```python
from build123d import *

# Parameters (mm, degrees)
BOSS_EXTRUDE1_DEPTH = 30
SKETCH2_R           = 2.5
CUT_EXTRUDE1_DEPTH  = 30


with BuildPart() as part:
    # Sketch1 → Boss-Extrude1 (new body)
    with BuildSketch(Plane.XY):
        with BuildLine():
            Line((0, 50), (0, 0))
            ThreePointArc((0, 0), (59.137285401, -30.145421821), (82.921098745, -92.115537233))
            Line((82.921098745, -92.115537233), (82.921098745, -120))
            Line((82.921098745, -120), (85.921098745, -120))
            Line((85.921098745, -120), (85.921098745, -92.115537233))
            ThreePointArc((85.921098745, -92.115537233), (62.264683971, -29.149857277), (3, 2.662090888))
            Line((3, 2.662090888), (3, 50))
            Line((3, 50), (0, 50))
        make_face()
    extrude(amount=BOSS_EXTRUDE1_DEPTH)

    # Sketch2 → Cut-Extrude1 (cut)
    with BuildSketch(Plane(origin=(85.921098745, 0, 0), x_dir=(0, 0, -1), z_dir=(1, 0, 0))):
        with Locations(Location((-15, -106.057768617, 0), (0, 0, 90))):
            Circle(SKETCH2_R)
    extrude(amount=-CUT_EXTRUDE1_DEPTH, mode=Mode.SUBTRACT)


solid = part.part
```
The model under review builds one solid part; all positions refer to its coordinate system, in mm. A direction names the side the tool comes from. Give positions to 0.01 mm unless a question says otherwise; leave off trailing zeros. Write each loop counter-clockwise with the first axis right and the second up, starting at its lowest first coordinate (ties: lowest second). Pieces come first, ordered by that corner, then holes. Notation, with made-up numbers: M 2.25,46.5 L 60.25,46.5 A17 cw 60.25,79.5 Z; hole C 15,-34 d9. An arc over 180 degrees is marked long. Write item = value, one per line. Start each with the question number.
Q1. For line 1 (X direction, y = 31, z = 6.25); line 2 (X direction, y = -107, z = 17.5); line 3 (Y direction, x = 27.5, z = 4.75), list the stretches that pass through material, from the lowest coordinate up.
Q2. We need section C-C (y = 38.5). State the section outline as (x, z) points, plus the area to 3 significant figures.
Q3. Machinability: for faces 1 (the face through (84, -120, 15)), 2 (the face through (3, 26, 15)), which of the approach directions +Z, -Z, +X, -X, +Y, -Y give a long, thin tool a straight path to every point of the face, cutting with its end or side? Answer none if there is none.
Q4. Mouldability with a two-part tool opening along Y and no side actions: class faces 3 (the face through (82.921, -103, 15)), 4 (the face through (84.442, -104.904, 12.782)), 5 (the face through (2, 50, 15)) as released by +Y, released by -Y, zero draft, split by the parting line, or undercut.
Q5. We need section A-A (z = 15). State the section outline as (x, y) points, plus the area to 3 significant figures.
Q6. We need section D-D (x = 59.5). State the section outline as (y, z) points, plus the area to 3 significant figures.
Q7. We need section B-B (z = 22.5). State the section outline as (x, y) points, plus the area to 3 significant figures.
Q8. Clearance check with flat-ended pins moving along their axes: pin 1 (8 mm diameter, centred on y = -48, z = 10, fed in from +X); pin 2 (2 mm diameter, centred on y = -12, z = 26, fed in from +X); pin 3 (3 mm diameter, centred on y = -9, z = 17.5, fed in from +X). State where each tip first meets the part, or that it passes through.
Result set:
q1.line_1 = 0 to 3
q1.line_2 = 82.92 to 85.92
q1.line_3 = -7.29 to -4.02
q2.outline = M 0,0 L 3,0 L 3,30 L 0,30 Z
q2.area = 90.0 mm2
q3.face_1 = +Z, -Z, +X, -X, -Y
q3.face_2 = +Z, -Z, +X, +Y
q4.face_3 = zero draft
q4.face_4 = undercut
q4.face_5 = released by +Y
q5.outline = M 0,0 A92.63 cw 82.92,-92.12 L 82.92,-103.56 L 85.92,-103.56 L 85.92,-92.12 A95.63 ccw 3,2.66 L 3,50 L 0,50 Z; M 82.92,-120 L 85.92,-120 L 85.92,-108.56 L 82.92,-108.56 Z
q5.area = 625 mm2
q6.outline = M -30.55,0 L -26.12,0 L -26.12,30 L -30.55,30 Z
q6.area = 133 mm2
q7.outline = M 0,0 A92.63 cw 82.92,-92.12 L 82.92,-120 L 85.92,-120 L 85.92,-92.12 A95.63 ccw 3,2.66 L 3,50 L 0,50 Z
q7.area = 640 mm2
q8.pin_1 = 77.1
q8.pin_2 = 44.01
q8.pin_3 = 40.13
